```python
from build123d import *

# Parameters (mm, degrees)
SKETCH1_W           = 130
SKETCH1_H           = 30
BOSS_EXTRUDE1_DEPTH = 5
BOSS_EXTRUDE3_DEPTH = 1.8
SKETCH6_W           = 40
SKETCH6_H           = 25
CUT_EXTRUDE2_DEPTH  = 2
SKETCH5_R           = 1.35
CUT_EXTRUDE3_DEPTH  = 6
SKETCH8_W           = 5
SKETCH8_H           = 30
BOSS_EXTRUDE4_DEPTH = 50
SKETCH9_R           = 10
CUT_EXTRUDE4_DEPTH  = 5
SKETCH10_W          = 30
SKETCH10_H          = 11.1
BOSS_EXTRUDE5_DEPTH = 30
SKETCH11_W          = 3.4
SKETCH11_H          = 30
CUT_EXTRUDE5_DEPTH  = 7
CUT_EXTRUDE6_REACH  = 173.828
SKETCH12_R          = 2.05
CUT_EXTRUDE7_DEPTH  = 5
SKETCH14_W          = 17.3
SKETCH14_H          = 30
CUT_EXTRUDE8_DEPTH  = 2
FILLET1_R           = 10
FILLET3_R           = 1
FILLET6_R           = 1


with BuildPart() as part:
    # Sketch1 → Boss-Extrude1 (new body)
    with BuildSketch(Plane(origin=(0, 0, 0), x_dir=(1, 0, 0), z_dir=(0, 1, 0))):
        with Locations((65, -15)):
            Rectangle(SKETCH1_W, SKETCH1_H)
    extrude(amount=BOSS_EXTRUDE1_DEPTH)

    # Sketch4 → Boss-Extrude3 (add)
    with BuildSketch(Plane.XZ):
        Polygon((63.1, 25), (66.9, 25), (66.9, 17), (66.9, 16.95), (67.95, 16.95), (74.95, 16.95), (74.95, 13.15), (66.95, 13.15), (66.9, 13.15), (66.9, 12.1), (66.9, 5.1), (63.1, 5.1), (63.1, 13.1), (63.1, 13.15), (62.05, 13.15), (55.05, 13.15), (55.05, 16.95), (63.05, 16.95), (63.1, 16.95), (63.1, 18), align=None)
    extrude(amount=BOSS_EXTRUDE3_DEPTH)

    # Sketch6 → Cut-Extrude2 (cut)
    with BuildSketch(Plane(origin=(0, 5, 0), x_dir=(1, 0, 0), z_dir=(0, 1, 0))):
        with Locations((65, -15)):
            Rectangle(SKETCH6_W, SKETCH6_H)
    extrude(amount=-CUT_EXTRUDE2_DEPTH, mode=Mode.SUBTRACT)

    # Sketch5 → Cut-Extrude3 (cut)
    with BuildSketch(Plane.XZ.offset(1.8)):
        with Locations(Location((65, 23, 0), (0, 0, 270))):
            Circle(SKETCH5_R)
        with Locations(Location((73, 15, 0), (0, 0, 270))):
            Circle(SKETCH5_R)
        with Locations(Location((57, 15, 0), (0, 0, 270))):
            Circle(SKETCH5_R)
        with Locations(Location((65, 7, 0), (0, 0, 270))):
            Circle(SKETCH5_R)
    extrude(amount=-CUT_EXTRUDE3_DEPTH, mode=Mode.SUBTRACT)

    # Sketch8 → Boss-Extrude4 (add)
    with BuildSketch(Plane(origin=(0, 5, 0), x_dir=(1, 0, 0), z_dir=(0, 1, 0))):
        with Locations((2.5, -15)):
            Rectangle(SKETCH8_W, SKETCH8_H)
        with Locations((127.5, -15)):
            Rectangle(SKETCH8_W, SKETCH8_H)
    extrude(amount=BOSS_EXTRUDE4_DEPTH)

    # Sketch9 → Cut-Extrude4 (cut)
    with BuildSketch(Plane(origin=(130, 0, 0), x_dir=(0, 0, -1), z_dir=(1, 0, 0))):
        with Locations((-15, 40)):
            Circle(SKETCH9_R)
    extrude(amount=-CUT_EXTRUDE4_DEPTH, mode=Mode.SUBTRACT)

    # Sketch10 → Boss-Extrude5 (add)
    with BuildSketch(Plane(origin=(130, 0, 0), x_dir=(0, 0, -1), z_dir=(1, 0, 0))):
        with Locations((-15, 13.55)):
            Rectangle(SKETCH10_W, SKETCH10_H)
    extrude(amount=BOSS_EXTRUDE5_DEPTH)

    # Sketch11 → Cut-Extrude5 (cut)
    with BuildSketch(Plane(origin=(0, 19.1, 0), x_dir=(1, 0, 0), z_dir=(0, 1, 0))):
        with Locations((131.7, -15)):
            Rectangle(SKETCH11_W, SKETCH11_H)
        with Locations((152.4, -15)):
            Rectangle(SKETCH11_W, SKETCH11_H)
    extrude(amount=-CUT_EXTRUDE5_DEPTH, mode=Mode.SUBTRACT)

    # Cut-Extrude6: up to this face of the body (flat: up to its plane)
    cut_extrude6_end = Plane(part.part.faces().sort_by_distance((130, 12.623489255, 15))[0])
    # Sketch12 → Cut-Extrude6 (cut, up to the picked face)
    with BuildSketch(Plane(origin=(160, 0, 0), x_dir=(0, 0, -1), z_dir=(1, 0, 0)), mode=Mode.PRIVATE) as cut_extrude6_sk1:
        with Locations((-15, 16)):
            Circle(SKETCH12_R)
    cut_extrude6_tool1 = split(extrude(cut_extrude6_sk1.sketch, amount=-CUT_EXTRUDE6_REACH, mode=Mode.PRIVATE), bisect_by=cut_extrude6_end, keep=Keep.BOTH, mode=Mode.PRIVATE)
    # Sketch12 → Cut-Extrude6 (cut, up to the picked face)
    with BuildSketch(Plane(origin=(160, 0, 0), x_dir=(0, 0, -1), z_dir=(1, 0, 0)), mode=Mode.PRIVATE) as cut_extrude6_sk2:
        with Locations((-21, 16)):
            Circle(SKETCH12_R)
    cut_extrude6_tool2 = split(extrude(cut_extrude6_sk2.sketch, amount=-CUT_EXTRUDE6_REACH, mode=Mode.PRIVATE), bisect_by=cut_extrude6_end, keep=Keep.BOTH, mode=Mode.PRIVATE)
    # Sketch12 → Cut-Extrude6 (cut, up to the picked face)
    with BuildSketch(Plane(origin=(160, 0, 0), x_dir=(0, 0, -1), z_dir=(1, 0, 0)), mode=Mode.PRIVATE) as cut_extrude6_sk3:
        with Locations((-9, 16)):
            Circle(SKETCH12_R)
    cut_extrude6_tool3 = split(extrude(cut_extrude6_sk3.sketch, amount=-CUT_EXTRUDE6_REACH, mode=Mode.PRIVATE), bisect_by=cut_extrude6_end, keep=Keep.BOTH, mode=Mode.PRIVATE)
    add(cut_extrude6_tool1.solids().sort_by(Axis((160, 16, 15), (-1, 0, 0)))[0], mode=Mode.SUBTRACT)
    add(cut_extrude6_tool2.solids().sort_by(Axis((160, 16, 21), (-1, 0, 0)))[0], mode=Mode.SUBTRACT)
    add(cut_extrude6_tool3.solids().sort_by(Axis((160, 16, 9), (-1, 0, 0)))[0], mode=Mode.SUBTRACT)

    # Sketch13 → Cut-Extrude7 (cut)
    with BuildSketch(Plane.ZY):
        with BuildLine():
            Line((9, 40), (9, 55))
            Line((9, 55), (21, 55))
            Line((21, 55), (21, 40))
            ThreePointArc((21, 40), (15, 34), (9, 40))
        make_face()
    extrude(amount=-CUT_EXTRUDE7_DEPTH, mode=Mode.SUBTRACT)

    # Sketch14 → Cut-Extrude8 (cut)
    with BuildSketch(Plane(origin=(0, 19.1, 0), x_dir=(1, 0, 0), z_dir=(0, 1, 0))):
        with Locations((142.05, -15)):
            Rectangle(SKETCH14_W, SKETCH14_H)
    extrude(amount=-CUT_EXTRUDE8_DEPTH, mode=Mode.SUBTRACT)

    # Fillet1
    # the kernel refuses this fillet: 10 mm, written as the material it takes off along each edge
    with BuildSketch(Plane(origin=(-24.874685928, 55, 0), x_dir=(0, -1, 0), z_dir=(1, 0, 0)), Plane(origin=(29.874685928, 55, 30), x_dir=(0, -1, 0), z_dir=(-1, 0, 0))) as fillet1_piece_1:
        with BuildLine():
            CenterArc((9.949874371, -10), FILLET1_R, 90, 84.260829523)
            Line((0, -9), (-0.198997487, -8.98))
            ThreePointArc((-0.198997487, -8.98), (-0.2, -4.5), (-0.2, 0))
            Line((-0.2, 0), (0, 0.2))
            Line((0, 0.2), (9.949874371, 0.2))
            Line((9.949874371, 0.2), (9.949874371, 0))
        make_face()
    extrude(amount=54.749371855, mode=Mode.SUBTRACT)
    with BuildSketch(Plane(origin=(155, 55, 0), x_dir=(0, -1, 0), z_dir=(-1, 0, 0)), Plane(origin=(100, 55, 30), x_dir=(0, -1, 0), z_dir=(1, 0, 0))) as fillet1_piece_2:
        with BuildLine():
            CenterArc((FILLET1_R, FILLET1_R), FILLET1_R, 180, 90)
            Line((0, FILLET1_R), (-FILLET1_R * 0.02, FILLET1_R))
            Line((-FILLET1_R * 0.02, FILLET1_R), (-FILLET1_R * 0.02, -FILLET1_R * 0.02))
            Line((-FILLET1_R * 0.02, -FILLET1_R * 0.02), (FILLET1_R, -FILLET1_R * 0.02))
            Line((FILLET1_R, -FILLET1_R * 0.02), (FILLET1_R, 0))
        make_face()
    extrude(amount=55, mode=Mode.SUBTRACT)

    # Fillet3
    fillet3_edges = [part.edges().sort_by_distance(p)[0] for p in [
        (2.5, 55, 9),
        (2.5, 55, 21),
    ]]
    fillet(fillet3_edges, radius=FILLET3_R)

    # Fillet6
    fillet6_edges = [part.edges().sort_by_distance(p)[0] for p in [
        (130, 40, 25),
        (125, 40, 25),
    ]]
    fillet(fillet6_edges, radius=FILLET6_R)


solid = part.part
```
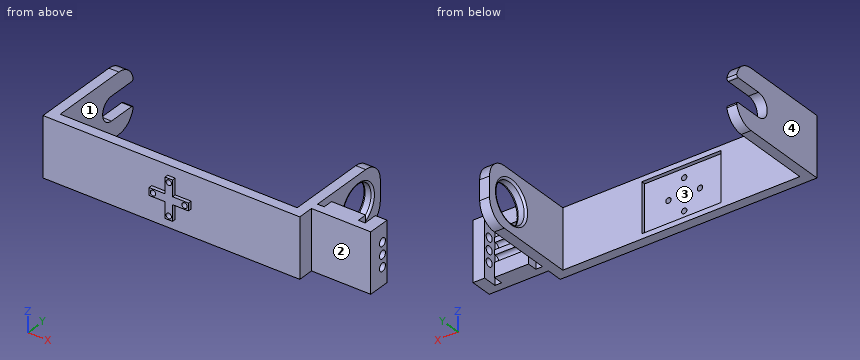
Design review of the part built by this model. Coordinates are the model's own, in mm. Face numbers are marked on the shaded views. A direction names the side the tool comes from. Give positions to 0.01 mm unless a question says otherwise; leave off trailing zeros. Order: outer loops, then holes, each group sorted by start corner. A loop starts at its lowest first (then second) coordinate and runs counter-clockwise, first axis right, second up. Notation, with made-up numbers: (-21.75, 78.5) - (7.25, 78.5) arc R16 ccw to (7.25, 100.5) - close; hole circle Ø9 at (-15, 44.5). An arc over 180 degrees is marked (long way). Use a Markdown table: item, result. Add a question column.
(1) Wall thickness on probe 1 along X at (y, z) = (16.5, 2.75); probe 2 along Z at (x, y) = (65, 1); probe 3 along X at (y, z) = (0.3, 23): over which ranges is each line inside the solid? List them lowest first. Write a range as [from, to].
(2) Add section A-A on y = 47.5. Give the number of separate pieces and of enclosed holes in the cut face, then the cut area to 3 significant figures.
(3) Clearance check with flat-ended pins moving along their axes: P1, Ø6, axis at x = 20.5, z = 4.5, coming from the -Y side; P2, Ø1.6, axis at x = 65, z = 23, coming from the +Y side; P3, Ø10, axis at y = 25, z = 18.5, coming from the +X side; P4, Ø1.4, axis at x = 72.5, y = -1, coming from the +Z side. State where each tip first meets the part, or that it passes through.
(4) Machinability: for the marked faces 1 and 2, which of the approach directions +Z, -Z, +X, -X, +Y, -Y give a long, thin tool a straight path to every point of the face, cutting with its end or side? Answer none if there is none.
(5) Mouldability with a two-part tool opening along Z and no side actions: class the marked faces 3 and 4 as +Z half, -Z half, draft (parallel to the pull), parting line (faces both ways), or undercut.
(6) Add section B-B on x = 43. Give the boundary of the cut face in (y, z), then the cut area to 3 significant figures.
Report:
| question | item | result |
|---|---|---|
| 1 | probe 1 | x = [0, 5], [125, 130], [133.4, 150.7], [154.1, 160] |
| 1 | probe 2 | z = [0, 5.65], [8.35, 21.65], [24.35, 30] |
| 1 | probe 3 | x = [0, 63.65], [66.35, 130] |
| 2 | separate pieces | 4 |
| 2 | enclosed holes | 0 |
| 2 | area | 166 mm² |
| 3 | P1 | stops at y = 0 |
| 3 | P2 | passes through |
| 3 | P3 | stops at x = 130 |
| 3 | P4 | stops at z = 16.95 |
| 4 | face 1 | +Z, -Z, +Y |
| 4 | face 2 | +Z, -Z, +X, -Y |
| 5 | face 3 | undercut |
| 5 | face 4 | draft |
| 6 | outline | (0, 0) - (5, 0) - (5, 30) - (0, 30) - close |
| 6 | area | 150 mm² |
